Verification items for this drawing (mm, ordinates from the low corner). A direction names the side the tool comes from. Round coordinates to 2 decimals unless told otherwise and drop trailing zeros. Loops run counter-clockwise (first coordinate to the right, second up) from the corner with the lowest first, then second, coordinate; pieces in that order, holes last. Notation, with made-up numbers: (81, -33.75) - (88, -33.75) arc R29 cw to (88, 0.25) - close; hole circle Ø8 at (-35, 73.5). An arc over 180 degrees is marked (long way). Answer in a Markdown table with one row per item. Add a question column.
(1) Access from +Z, -Z, +X, -X, +Y, -Y to the whole of each face (thin tool, end or side, straight path). Record for the marked faces 1 and 2.
(2) Mould release check, pull along X, two halves, no side actions. Record for the marked faces 3, 4 and 5: +X half, -X half, draft (parallel to the pull), parting line (faces both ways), or undercut.
(3) Gauge pin test, flat ends, axial feed: pin 1 (4 mm diameter, centred on x = 72, y = 35, fed in from -Z); pin 2 (3 mm diameter, centred on y = 25, z = 94.58, fed in from +X); pin 3 (6 mm diameter, centred on x = 105, y = 30, fed in from +Z); pin 4 (6.5 mm diameter, centred on y = 25, z = 154.06, fed in from +X). Record the tip position at first contact, or that the pin passes through.
(4) Cross-section at D-D on x = 18. Enter the section's corners in (y, z) (1 decimal), then the cut area to 3 significant figures.
(5) Thickness scan on line 1 along Z through (x, y) = (12, 25) (1 decimal); line 2 along Z through (x, y) = (11, 25) (1 decimal); line 3 along X through (y, z) = (40.5, 55.5) (1 decimal). Record the ranges inside material, lowest first.
(6) Cross-section at C-C on z = 59. Enter the section's corners in (x, y) (1 decimal).
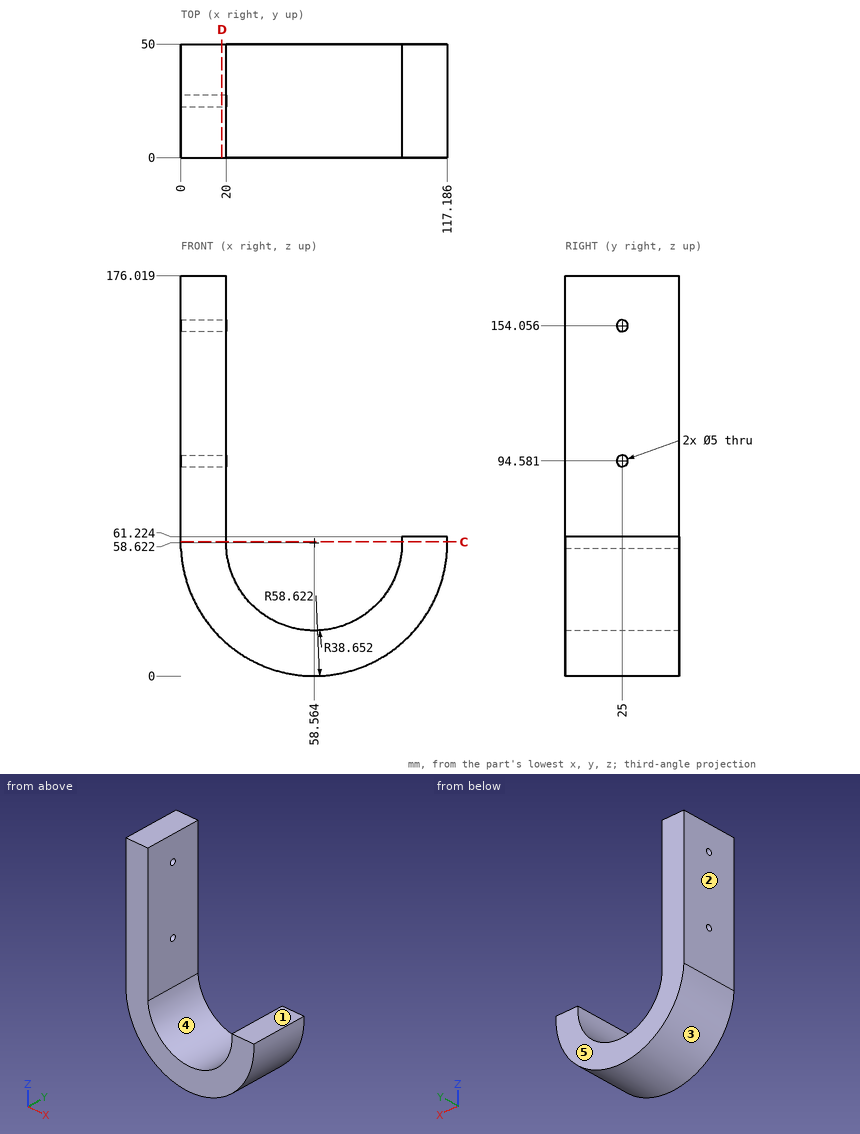
Answers:
| question | item | result |
|---|---|---|
| 1 | face 1 | +Z, +X, +Y, -Y |
| 1 | face 2 | +Z, -Z, -X, +Y, -Y |
| 2 | face 3 | parting line |
| 2 | face 4 | undercut |
| 2 | face 5 | draft |
| 3 | pin 1 | stops at z = 1.13 |
| 3 | pin 2 | passes through |
| 3 | pin 3 | stops at z = 61.22 |
| 3 | pin 4 | stops at x = 20 |
| 4 | outline | (0, 16.3) - (50, 16.3) - (50, 176) - (0, 176) - close; hole circle Ø5 at (25, 94.6); hole circle Ø5 at (25, 154.1) |
| 4 | area | 7,950 mm^2 |
| 5 | line 1 | z = 23 to 92.1, 97.1 to 151.6, 156.6 to 176 |
| 5 | line 2 | z = 24.4 to 92.1, 97.1 to 151.6, 156.6 to 176 |
| 5 | line 3 | x = 0 to 20, 97.1 to 117.1 |
| 6 | outline | (0, 0) - (20, 0) - (20, 50) - (0, 50) - close; (97.2, 0) - (117.2, 0) - (117.2, 50) - (97.2, 50) - close |
